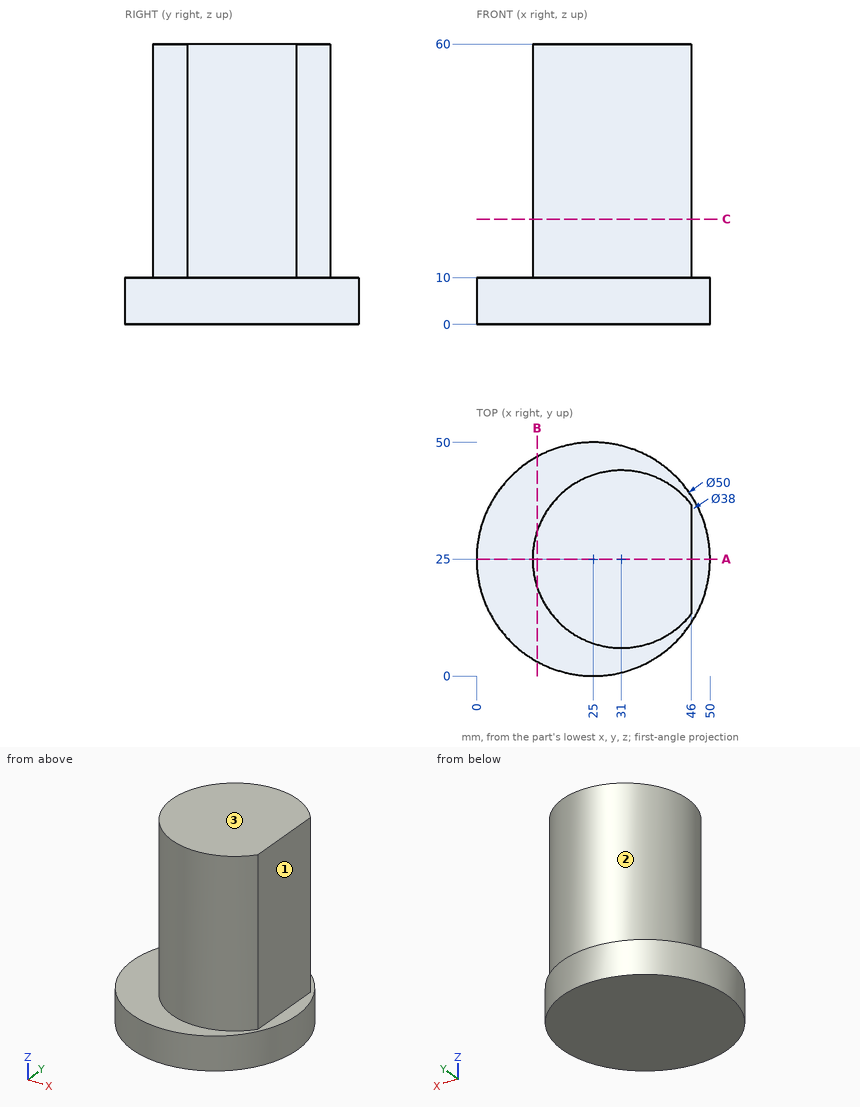
Check sheet for the drawn part. Datum: minimum x, y, z corner. Units: mm. A direction names the side the tool comes from. Round coordinates to 2 decimals unless told otherwise and drop trailing zeros. Order: outer loops, then holes, each group sorted by start corner. A loop starts at its lowest first (then second) coordinate and runs counter-clockwise, first axis right, second up. Notation, with made-up numbers: (49.5, -24) -> (61.5, -24) arc R19 ccw to (61.5, 5) -> close; hole circle Ø7 at (-0.5, -39.75). An arc over 180 degrees is marked (long way). Return JSON: item names as keys, results as strings. Group by question number.
Q1. Gauge pin test, flat ends, axial feed: pin 1 (12 mm diameter, centred on x = 24, z = 15.5, fed in from -Y); pin 2 (10 mm diameter, centred on x = 13, z = 8.5, fed in from +Y); pin 3 (4 mm diameter, centred on x = 10, y = 43.5, fed in from +Z). Record the tip position at first contact, or that the pin passes through.
Q2. Section check A-A, the plane y = 25. Record the boundary of the cut face in (x, z).
Q3. Material ranges on probe 1 along Z at (x, y) = (7.5, 35); probe 2 along Y at (x, z) = (31.5, 37); probe 3 along X at (y, z) = (18, 14.5), recorded low to high. Write a range as from..to.
Q4. Section check C-C, the plane z = 22.5. Record the boundary of the cut face in (x, y).
Q5. Section check B-B, the plane x = 13. Record the boundary of the cut face in (y, z), plus the area to 3 significant figures.
Q6. Tool access check on the marked faces 1, 2 and 3. Record the directions out of +Z, -Z, +X, -X, +Y, -Y that give a thin tool (end or side, any length) a straight path to the whole face; none if there is none.
Numbers:
{
 "1": {"pin 1": "y = 0", "pin 2": "y = 49", "pin 3": "z = 10"},
 "2": {"outline": "(0, 0) -> (50, 0) -> (50, 10) -> (46, 10) -> (46, 60) -> (12, 60) -> (12, 10) -> (0, 10) -> close"},
 "3": {"probe 1": "0..10", "probe 2": "6.01..43.99", "probe 3": "13.34..46"},
 "4": {"outline": "(46, 13.34) -> (46, 36.66) arc R19 ccw (long way) to start"},
 "5": {"outline": "(3.07, 0) -> (46.93, 0) -> (46.93, 10) -> (31.08, 10) -> (31.08, 60) -> (18.92, 60) -> (18.92, 10) -> (3.07, 10) -> close", "area": "1,050 mm^2"},
 "6": {"face 1": "+Z, +X, +Y, -Y", "face 2": "+Z", "face 3": "+Z, +X, -X, +Y, -Y"}
}
